Work out the finished part from the listing and answer in its coordinate system (mm). A direction names the side the tool comes from. Round coordinates to 2 decimals unless told otherwise and drop trailing zeros. Order: outer loops, then holes, each group sorted by start corner. A loop starts at its lowest first (then second) coordinate and runs counter-clockwise, first axis right, second up. Notation, with made-up numbers: (25, 62) -> (45, 62) arc R12 ccw to (45, 74) -> close; hole circle Ø2 at (-10, 18.5). An arc over 180 degrees is marked (long way). Use a Markdown table: item, result. Add a question column.
Item 1: A cutting plane is placed at C-C, the plane x = -11. Determine the outline of the cut face in (y, z).
Item 2: For a pull along X with two mould halves and no side action, classify faces 1 (the flat face through (-2, 0, 0)), 2 (the flat face through (16.885, 0, 3)), 3 (the flat face through (-17.798, 0, 4)) as +X half, -X half, draft (parallel to the pull), parting line (faces both ways), or undercut.
Item 3: A tool of negligible diameter and unlimited length cuts with its end or side. For faces 4 (the flat face through (-1, -26.842, 3)), 5 (the flat face through (-1, -24.842, 4)), from which of +Z, -Z, +X, -X, +Y, -Y can it reach the whole face along a straight path? Write none if from no direction.
Item 4: Flat-ended cylindrical pins translate along their axes: P1, Ø8, axis at x = -13, y = -2, coming from the +Z side; P2, Ø4, axis at x = -1.46, y = -20.8, coming from the -Z side. Find the tip coordinate at first contact, or state that the pin passes through.
Item 5: A cutting plane is placed at B-B, the plane z = 4.5. Determine the outline of the cut face in (x, y), plus the area to 3 significant figures.
Item 6: A cutting plane is placed at D-D, the plane y = -9. Determine the outline of the cut face in (x, z).
Item 7: A cutting plane is placed at A-A, the plane y = -20.8. Determine the outline of the cut face in (x, z), plus the area to 3 significant figures.
Item 8: Find the intervals of material crossed by L1, parallel to X at y = 4, z = 3; L2, parallel to Y at x = -8, z = 5.6; L3, parallel to Y at x = -0.5, z = 1.05, in increasing order. Write a range as [from, to].
Autodesk Inventor part; units mm, degrees
ref_plane "YZ Plane" through (0, 0, 0) normal (1, 0, 0) x (0, 1, 0)
ref_plane "XZ Plane" through (0, 0, 0) normal (0, 1, 0) x (-1, 0, 0)
ref_plane "XY Plane" through (0, 0, 0) normal (0, 0, 1) x (1, 0, 0)
sketch "Sketch1" plane through (0, 0, 0) normal (0, 0, 1) x (1, 0, 0)
  circle A0 centre (-1.4563, 20.8) radius 1.5
  circle A1 centre (-1.4563, -20.8) radius 1.5
  arc A2 (-17.4563, 26.8416) -> (-19.7979, 24.5) centre (-17.4563, 24.5) ccw
  line L0 (-19.7979, -24.5) -> (-19.7979, 24.5)
  arc A3 (-19.7979, -24.5) -> (-17.4563, -26.8416) centre (-17.4563, -24.5) ccw
  line L1 (14.5437, -26.8416) -> (-17.4563, -26.8416)
  arc A4 (14.5437, -26.8416) -> (16.8852, -24.5) centre (14.5437, -24.5) ccw
  line L2 (16.8852, 24.5) -> (16.8852, -24.5)
  arc A5 (16.8852, 24.5) -> (14.5437, 26.8416) centre (14.5437, 24.5) ccw
  line L3 (-17.4563, 26.8416) -> (14.5437, 26.8416)
  arc A6 (14.8852, 24.5) -> (14.5437, 24.8416) centre (14.5437, 24.5) ccw
  line L4 (14.8852, 24.5) -> (14.8852, -24.5)
  arc A7 (14.5437, -24.8416) -> (14.8852, -24.5) centre (14.5437, -24.5) ccw
  line L5 (14.5437, -24.8416) -> (-17.4563, -24.8416)
  arc A8 (-17.7979, -24.5) -> (-17.4563, -24.8416) centre (-17.4563, -24.5) ccw
  line L6 (-17.7979, -24.5) -> (-17.7979, 24.5)
  arc A9 (-17.4563, 24.8416) -> (-17.7979, 24.5) centre (-17.4563, 24.5) ccw
  line L7 (-17.4563, 24.8416) -> (14.5437, 24.8416)
  point P0 (0, 0)
  point P1 (0, 0)
  dimension "d0" = 2
extrude "Extrusion1" add sketch "Sketch1" along normal blind 6 contours L3 A5 L2 A4 L1 A3 L0 A2
extrude "Extrusion2" add sketch "Sketch1" along normal blind 2.5 contours L4 A7 L5 A8 L6 A9 L7 A6
sketch "Sketch2" plane through (0, 0, 2.5) normal (0, 0, 1) x (1, 0, 0)
  circle A0 centre (-1.4563, -20.8) radius 1.5
  circle A1 centre (-1.4563, 20.8) radius 1.5
  line L0 (14.8852, 24.5) -> (14.8852, -24.5)
  arc A2 (14.8852, 24.5) -> (14.5437, 24.8416) centre (14.5437, 24.5) ccw
  line L1 (-17.4563, 24.8416) -> (14.5437, 24.8416)
  arc A3 (-17.4563, 24.8416) -> (-17.7979, 24.5) centre (-17.4563, 24.5) ccw
  line L2 (-17.7979, -24.5) -> (-17.7979, 24.5)
  arc A4 (-17.7979, -24.5) -> (-17.4563, -24.8416) centre (-17.4563, -24.5) ccw
  line L3 (14.5437, -24.8416) -> (-17.4563, -24.8416)
  arc A5 (14.5437, -24.8416) -> (14.8852, -24.5) centre (14.5437, -24.5) ccw
  point P0 (0, 0)
chamfer "Chamfer1" distance 1 angle 45 2 edges at (-2.9563, -20.8, 0) (-2.9563, 20.8, 0)
properties part number "Tapa"
Reported:
| question | item | result |
|---|---|---|
| 1 | outline | (-26.84, 0) -> (26.84, 0) -> (26.84, 6) -> (24.84, 6) -> (24.84, 2.5) -> (-24.84, 2.5) -> (-24.84, 6) -> (-26.84, 6) -> close |
| 2 | face 1 | draft |
| 2 | face 2 | +X half |
| 2 | face 3 | undercut |
| 3 | face 4 | +Z, -Z, +X, -X, -Y |
| 3 | face 5 | +Z |
| 4 | P1 | z = 2.5 |
| 4 | P2 | z = 0.5 |
| 5 | outline | (-19.8, -24.5) arc R2.34 ccw to (-17.46, -26.84) -> (14.54, -26.84) arc R2.34 ccw to (16.89, -24.5) -> (16.89, 24.5) arc R2.34 ccw to (14.54, 26.84) -> (-17.46, 26.84) arc R2.34 ccw to (-19.8, 24.5) -> close; hole (-17.8, -24.5) arc R0.34 ccw to (-17.46, -24.84) -> (14.54, -24.84) arc R0.34 ccw to (14.89, -24.5) -> (14.89, 24.5) arc R0.34 ccw to (14.54, 24.84) -> (-17.46, 24.84) arc R0.34 ccw to (-17.8, 24.5) -> close |
| 5 | area | 341 mm² |
| 6 | outline | (-19.8, 0) -> (16.89, 0) -> (16.89, 6) -> (14.89, 6) -> (14.89, 2.5) -> (-17.8, 2.5) -> (-17.8, 6) -> (-19.8, 6) -> close |
| 7 | outline | (-19.8, 0) -> (-3.96, 0) -> (-2.96, 1) -> (-2.96, 2.5) -> (-17.8, 2.5) -> (-17.8, 6) -> (-19.8, 6) -> close; (0.04, 1) -> (1.04, 0) -> (16.89, 0) -> (16.89, 6) -> (14.89, 6) -> (14.89, 2.5) -> (0.04, 2.5) -> close |
| 7 | area | 97.2 mm² |
| 8 | L1 | [-19.8, -17.8], [14.89, 16.89] |
| 8 | L2 | [-26.84, -24.84], [24.84, 26.84] |
| 8 | L3 | [-26.84, -21.96], [-19.64, 19.64], [21.96, 26.84] |
